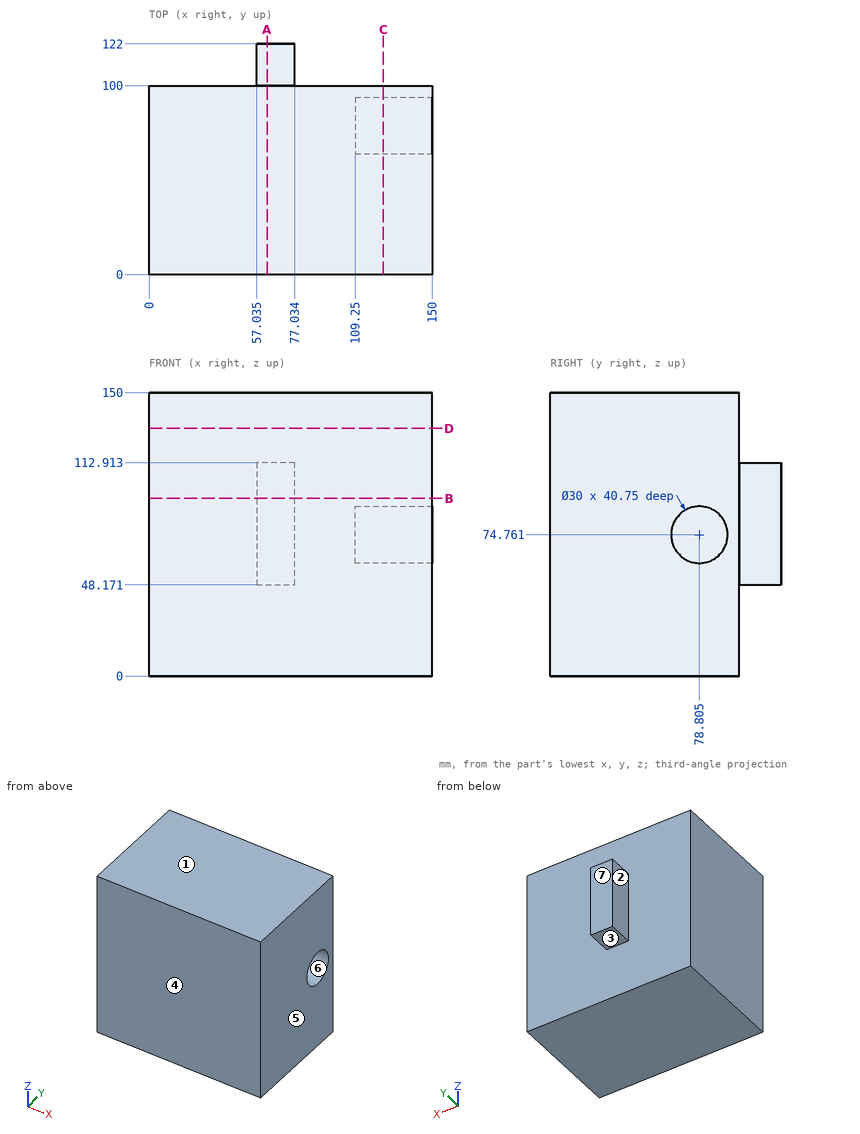
Print and shaded views of the part. All mm, measured from the part's lowest x, y and z. A direction names the side the tool comes from. Coordinates: 2 decimals unless noted, no trailing zeros. Order: outer loops, then holes, each group sorted by start corner. A loop starts at its lowest first (then second) coordinate and runs counter-clockwise, first axis right, second up. Notation, with made-up numbers: (48.25, -1) -> (60.25, -1) arc R24 cw to (60.25, 9) -> close; hole circle Ø7 at (-22.75, 27.5). An arc over 180 degrees is marked (long way). Answer as a JSON object with one key per item and string values. Group by question number.
1) Cut at B-B, the plane z = 94. Write the cut outline in (x, y) (1 decimal), then the cut area to 3 significant figures.
2) Pull direction Y, two halves, no side cores. Call the marked faces 4, 5, 6 and 7: +Y half, -Y half, draft (parallel to the pull), parting line (faces both ways), or undercut.
3) Which spindle directions (+Z, -Z, +X, -X, +Y, -Y) get a long thin tool onto all of the face, cutting with end or side? Do the marked faces 1, 2 and 3. Say none if no direction does.
4) Cut at D-D, the plane z = 131. Write the cut outline in (x, y), then the cut area to 3 significant figures.
5) Flat gauge pins, fed straight in: pin 1 (12 mm diameter, centred on x = 50, z = 123, fed in from +Y); pin 2 (6 mm diameter, centred on x = 66, y = 110, fed in from +Z); pin 3 (15 mm diameter, centred on y = 76, z = 70.5, fed in from +X). Where does each tip first touch, or does it go through?
6) Cut at A-A, the plane x = 62.5. Write the cut outline in (y, z).
7) Cut at C-C, the plane x = 124. Write the cut outline in (y, z) (1 decimal).
8) Drill centre lines: L1, parallel to X at y = 115, z = 49 (1 decimal); L2, parallel to Y at x = 44.5, z = 133.5; L3, parallel to Z at x = 126, y = 90 (1 decimal). Where is each one in solid material? Low to high.
Check values:
{
 "1": {"outline": "(0, 0) -> (150, 0) -> (150, 100) -> (77, 100) -> (77, 122) -> (57, 122) -> (57, 100) -> (0, 100) -> close", "area": "15,400 mm²"},
 "2": {"face 4": "-Y half", "face 5": "draft", "face 6": "undercut", "face 7": "+Y half"},
 "3": {"face 1": "+Z, +X, -X, +Y, -Y", "face 2": "+Z, -Z, -X, +Y", "face 3": "-Z, +X, -X, +Y"},
 "4": {"outline": "(0, 0) -> (150, 0) -> (150, 100) -> (0, 100) -> close", "area": "15,000 mm²"},
 "5": {"pin 1": "stops at y = 100", "pin 2": "stops at z = 112.91", "pin 3": "stops at x = 109.25"},
 "6": {"outline": "(0, 0) -> (100, 0) -> (100, 48.17) -> (122, 48.17) -> (122, 112.91) -> (100, 112.91) -> (100, 150) -> (0, 150) -> close"},
 "7": {"outline": "(0, 0) -> (100, 0) -> (100, 150) -> (0, 150) -> close; hole circle Ø30 at (78.8, 74.8)"},
 "8": {"L1": "x = 57 to 77", "L2": "y = 0 to 100", "L3": "z = 0 to 64.8, 84.7 to 150"}
}
